Autodesk Inventor part; units mm, degrees
ref_plane "YZ Plane" through (0, 0, 0) normal (1, 0, 0) x (0, 1, 0)
ref_plane "XZ Plane" through (0, 0, 0) normal (0, 1, 0) x (-1, 0, 0)
ref_plane "XY Plane" through (0, 0, 0) normal (0, 0, 1) x (1, 0, 0)
sketch "Sketch1" plane through (0, 0, 0) normal (0, 0, 1) x (1, 0, 0)
  line L0 (0, 0) -> (19.1, 0)
  line L1 (19.1, 0) -> (19.1, 19.1)
  line L2 (19.1, 19.1) -> (0, 19.1)
  line L3 (0, 19.1) -> (0, 0)
  dimension "d0" = 19.1
  dimension "d1" = 19.1
extrude "Extrusion1" add sketch "Sketch1" along normal blind 8.67
sketch "Sketch2" plane through (19.1, 0, 0) normal (1, 0, 0) x (0, 0, -1)
  line L0 (0, 0) -> (0, 19.1)
  line L1 (0, 19.1) -> (-8.67, 19.1)
  line L2 (-8.67, 0) -> (-8.67, 19.1)
  line L3 (0, 0) -> (-8.67, 0)
  line L4 (0, 0) -> (0, 19.1) construction
  line L5 (0, 9.55) -> (-11, 9.55) construction
  line L6 (-11, 9.55) -> (-11, 16.3311) construction
  circle A0 centre (-10, 9.55) radius 1
  circle A1 centre (-10, 9.55) radius 2
  point P0 (-8.67, 11.0437)
  point P1 (-8.67, 8.0563)
  dimension "d4" = 11
  dimension "d5" = 2
  dimension "d6" = 4
extrude "Extrusion2" add sketch "Sketch2" against normal up to surface (19.1 mm away) contours A1 L2 picked at (-8.78, 9.55)
sketch "Sketch3" plane through (0, 0, 8.67) normal (0, 0, 1) x (1, 0, 0)
  line L0 (0, 11.0437) -> (19.1, 11.0437)
  line L1 (19.1, 11.0437) -> (19.1, 19.1)
  line L2 (19.1, 19.1) -> (0, 19.1)
  line L3 (0, 19.1) -> (0, 11.0437)
  line L4 (19.1, 8.0563) -> (0, 8.0563)
  line L5 (0, 8.0563) -> (0, 0)
  line L6 (0, 0) -> (19.1, 0)
  line L7 (19.1, 0) -> (19.1, 8.0563)
  line L8 (19.1, 19.1) -> (0, 19.1) construction
  line L9 (9.55, 19.1) -> (9.55, 0) construction
  circle A0 centre (9.55, 9.55) radius 7
  dimension "d9" = 14
extrude "Extrusion3" add sketch "Sketch3" along normal blind 9.93 contours A0 L0 | L0 A0 L4 | L4 A0
sketch "Sketch4" plane through (0, 0, 0) normal (0, -1, 0) x (1, 0, 0)
  line L0 (0, 0) -> (19.1, 0)
  line L1 (16.55, 18.6) -> (2.55, 18.6)
  dimension "d12" = 18.6
sketch "Sketch5" plane through (19.1, 0, 0) normal (1, 0, 0) x (0, 0, -1)
  line L0 (0, 0) -> (0, 19.1)
  line L1 (0, 9.55) -> (-151.3307, 9.55)
  line L2 (-18.6, 16.55) -> (-18.6, 2.55)
  line L3 (-18.6, 16.55) -> (-47.9586, 84.0702)
  line L4 (-18.6, 2.55) -> (-41.5927, -50.3296)
  dimension "d13" = 133
sketch "Sketch6" plane through (0, 19.1, 0) normal (0, 1, 0) x (1, 0, 0)
  line L0 (19.1, 0) -> (0, 0)
  line L1 (0, 0) -> (0, -8.67)
  line L2 (19.1, -8.67) -> (0, -8.67)
  line L3 (19.1, 0) -> (19.1, -8.67)
  line L4 (2.55, -18.6) -> (16.55, -18.6)
  line L5 (9.55, -18.6) -> (-223.0708, -119.7464)
  line L6 (9.55, -18.6) -> (332.284, -158.9287)
  line L7 (9.55, -18.6) -> (9.55, 0)
  line L8 (0, 0) -> (19.1, 0)
  dimension "d14" = 133
ref_plane "Work Plane1" through (0, 9.55, 0) normal (0, 1, 0) x (1, 0, 0)
sketch "Sketch7" plane through (0, 9.55, 0) normal (0, 1, 0) x (1, 0, 0)
  line L0 (9.55, -18.6) -> (-223.0708, -119.7464)
  line L1 (9.55, -18.6) -> (332.284, -158.9287)
  point P0 (0, 0)
properties part number "HDzero micro dummy"
Could you check a few things on this model? Use its own coordinates, in mm. A direction names the side the tool comes from. Round coordinates to 2 decimals unless told otherwise and drop trailing zeros. Loops run counter-clockwise (first coordinate to the right, second up) from the corner with the lowest first, then second, coordinate; pieces in that order, holes last. Notation, with made-up numbers: (40.5, -21.75) - (80.5, -21.75) arc R22 cw to (80.5, -7.75) - close; hole circle Ø4 at (73, 80). An arc over 180 degrees is marked (long way). Answer as CSV lines item,"result".
1. I want a section at D-D on x = 3.75. List the corners of the cut face in (y, z) for me, then the cut area to 3 significant figures.
Filled in:
outline,"(0, 0) - (19.1, 0) - (19.1, 8.67) - (13.47, 8.67) - (13.47, 18.6) - (5.63, 18.6) - (5.63, 8.67) - (0, 8.67) - close"
area,"243 mm^2"
2. Please list where these lines run through material, in increasing order: line 1 along Y through (x, z) = (18, 10); line 2 along Z through (x, y) = (0.65, 9.55); line 3 along Y through (x, z) = (9.75, 17.5). Write a range as [from, to].
Filled in:
line 1,"y = [7.55, 8.55], [10.55, 11.55]"
line 2,"z = [0, 9], [11, 12]"
line 3,"y = [2.55, 16.55]"
3. I want a section at B-B on y = 9.55. List the corners of the cut face in (x, z) for me, then the cut area to 3 significant figures.
Filled in:
outline,"(0, 0) - (19.1, 0) - (19.1, 9) - (16.55, 9) - (16.55, 11) - (19.1, 11) - (19.1, 12) - (16.55, 12) - (16.55, 18.6) - (2.55, 18.6) - (2.55, 12) - (0, 12) - (0, 11) - (2.55, 11) - (2.55, 9) - (0, 9) - close"
area,"311 mm^2"
4. For pin 1 Ø1.2 at (y, z) = (9.55, 10) entering from -X; pin 2 Ø3 at (x, z) = (13.5, 16) entering from -Y; pin 3 Ø1 at (x, z) = (4, 10) entering from -Y, each with a flat end and sliding along its axis, tell me the tip position at first contact or that it passes through.
Filled in:
pin 1,"stops at x = 2.55"
pin 2,"stops at y = 2.99"
pin 3,"stops at y = 4.7"
5. I want a section at C-C on z = 14.25. List the corners of the cut face in (x, y) for me.
Filled in:
outline,"circle Ø14 at (9.55, 9.55)"
6. We'd pull the mould along Y, two halves only. Please class faces 3 (the face through (10, 19.1, 4)), 4 (the face through (19.1, 9, 5)), 5 (the face through (17.81, 8.94, 10.79)): +Y half, -Y half, draft (parallel to the pull), parting line (faces both ways), or undercut.
Filled in:
face 3,"+Y half"
face 4,"draft"
face 5,"undercut"
7. On a 3-axis mill with a long thin cutter (end or side, diameter ignored), from which of +Z, -Z, +X, -X, +Y, -Y can I reach the whole of each face in a straight line? I mean faces 1 (the face through (1.33, 8.94, 10.79)), 2 (the face through (9, 10, 18.6)). Say none if no direction works.
Filled in:
face 1,"-X"
face 2,"+Z, +X, -X, +Y, -Y"
8. I want a section at A-A on x = 9.55. List the corners of the cut face in (y, z) for me, then the cut area to 3 significant figures.
Filled in:
outline,"(0, 0) - (19.1, 0) - (19.1, 8.67) - (16.55, 8.67) - (16.55, 18.6) - (2.55, 18.6) - (2.55, 8.67) - (0, 8.67) - close"
area,"305 mm^2"
